```python
from build123d import *

# Parameters (mm, degrees)
SKETCH_1_R          = 7.5
EXTRUDE_1_DEPTH     = 215
CUT_EXTRUDE_1_DEPTH = 2.5
SKETCH_3_R          = 4
EXTRUDE_2_DEPTH     = 20


with BuildPart() as part:
    # 草图1 → 凸台-拉伸1 (new, symmetric)
    with BuildSketch(Plane.XY):
        Circle(SKETCH_1_R)
    extrude(amount=EXTRUDE_1_DEPTH, both=True)

    # 草图2 → 切除-拉伸1 (cut)
    with BuildSketch(Plane(origin=(0, 7.5, 0), x_dir=(1, 0, 0), z_dir=(0, 1, 0))):
        with BuildLine():
            Line((2.5, -152.5), (2.5, -172.5))
            ThreePointArc((2.5, -172.5), (0, -175), (-2.5, -172.5))
            Line((-2.5, -172.5), (-2.5, -152.5))
            ThreePointArc((-2.5, -152.5), (0, -150), (2.5, -152.5))
        make_face()
        with BuildLine():
            Line((2.5, 152.5), (2.5, 172.5))
            ThreePointArc((2.5, 172.5), (0, 175), (-2.5, 172.5))
            Line((-2.5, 172.5), (-2.5, 152.5))
            ThreePointArc((-2.5, 152.5), (0, 150), (2.5, 152.5))
        make_face()
    extrude(amount=-CUT_EXTRUDE_1_DEPTH, mode=Mode.SUBTRACT)

    # 草图3 → 凸台-拉伸2 (add)
    with BuildSketch(Plane.XY.offset(215)):
        Circle(SKETCH_3_R)
    extrude_2 = extrude(amount=EXTRUDE_2_DEPTH)

    # 镜向1: 凸台-拉伸2 across plane
    add(extrude_2.mirror(Plane.XY))


solid = part.part
```
Check sheet for the modelled part. Datum: model origin and axes. Units: mm. A direction names the side the tool comes from. Give positions to 0.01 mm unless a question says otherwise; leave off trailing zeros. Order: outer loops, then holes, each group sorted by start corner. A loop starts at its lowest first (then second) coordinate and runs counter-clockwise, first axis right, second up. Notation, with made-up numbers: (43.25, -15.75) -> (98.25, -15.75) arc R25 ccw to (98.25, 8.25) -> close; hole circle Ø3 at (89, 6.25). An arc over 180 degrees is marked (long way). Use CSV: the item, a comma, the result in double quotes. Start each with the question number.
1) Go/stop test with flat-tipped pins: P1, Ø5, axis at x = 4, z = 132.5, coming from the -Y side; P2, Ø1.5, axis at x = 1, y = -6, coming from the -Z side; P3, Ø8, axis at y = 6, z = -166, coming from the +X side. Record where each tip stops, or that it passes through.
2) Mould release check, pull along X, two halves, no side actions. Record for faces 1 (the face through (0, 0, 235)), 2 (the face through (-0.867, -3.905, -224.86)): released by +X, released by -X, zero draft, split by the parting line, or undercut.
3) Sectioned sample at B-B, the plane z = -166. Record the boundary of the cut face in (x, y).
4) Material ranges on line 1 (Z direction, x = 3, y = 6.75); line 2 (X direction, y = -0.75, z = -104.5); line 3 (Y direction, x = 0.5, z = 7.5), recorded low to high. Write a range as from..to.
5) Sectioned sample at A-A, the plane y = 0. Record the boundary of the cut face in (x, z), plus the area to 3 significant figures.
6) Set-up check for faces 3 (the face through (-0.867, -3.905, 224.86)), 4 (the face through (-7.493, 0.33, 3.01)), 5 (the face through (3, -3, -215)): record each of +Z, -Z, +X, -X, +Y, -Y from which the full face is reachable in a straight line by a thin tool's end or side.
Recorded:
1,P1,"y = -7.35"
1,P2,"z = -215"
1,P3,"x = 7.23"
2,face 1,"zero draft"
2,face 2,"split by the parting line"
3,outline,"(-2.5, 5) -> (-2.5, 7.07) arc R7.5 ccw (long way) to (2.5, 7.07) -> (2.5, 5) -> close"
4,line 1,"-215..215"
4,line 2,"-7.46..7.46"
4,line 3,"-7.48..7.48"
5,outline,"(-7.5, -215) -> (-4, -215) -> (-4, -235) -> (4, -235) -> (4, -215) -> (7.5, -215) -> (7.5, 215) -> (4, 215) -> (4, 235) -> (-4, 235) -> (-4, 215) -> (-7.5, 215) -> close"
5,area,"6,770 mm2"
6,face 3,"+Z"
6,face 4,"+Z, -Z"
6,face 5,"-Z"
